Here's the drawing with two shaded views (mm, measured from the low corner). I have some questions. A direction names the side the tool comes from. Coordinates: 2 decimals unless noted, no trailing zeros. Order: outer loops, then holes, each group sorted by start corner. A loop starts at its lowest first (then second) coordinate and runs counter-clockwise, first axis right, second up. Notation, with made-up numbers: (-22.75, 20) -> (19.25, 20) arc R21 ccw to (19.25, 51) -> close; hole circle Ø6 at (-38, 88). An arc over 180 degrees is marked (long way). Return JSON: item names as keys, results as strings. Group by question number.
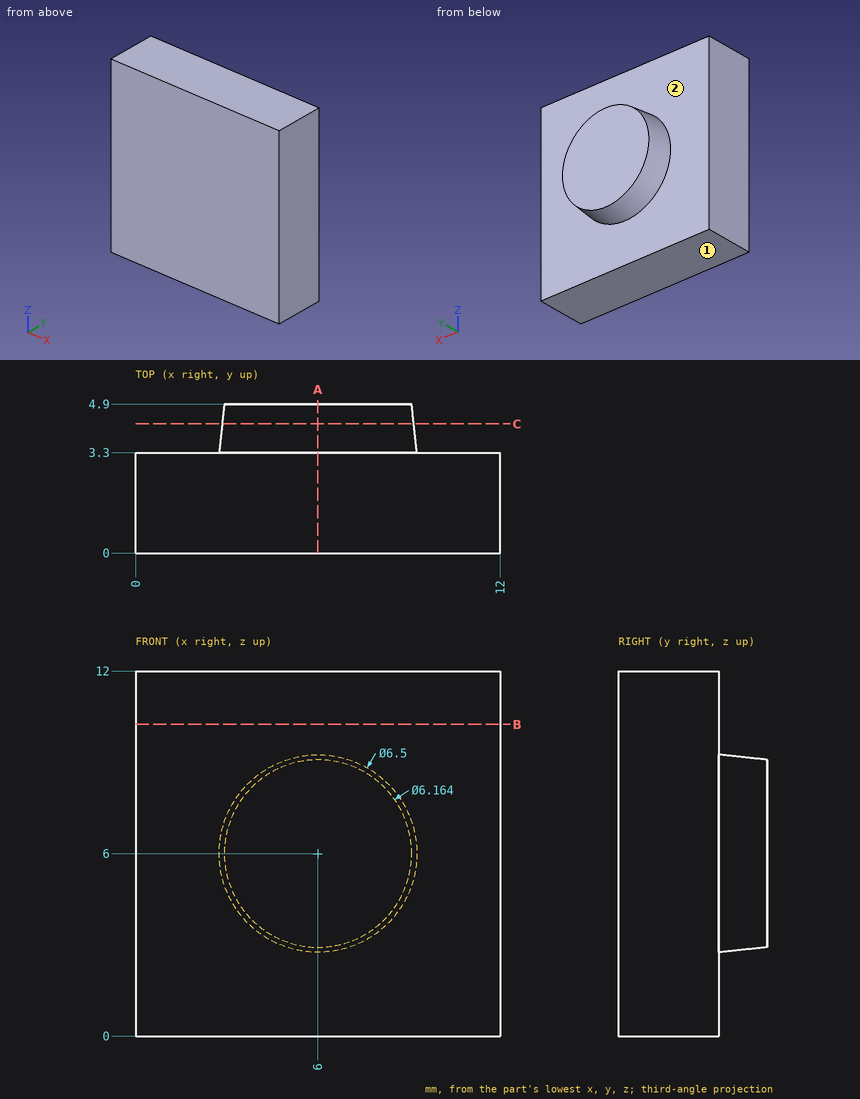
Q1. On a 3-axis mill with a long thin cutter (end or side, diameter ignored), from which of +Z, -Z, +X, -X, +Y, -Y can I reach the whole of each face in a straight line? I mean the marked faces 1 and 2. Say none if no direction works.
Q2. I want a section at B-B on z = 10.25. Please give me the cut outline in (x, y).
Q3. I want a section at C-C on y = 4.25. Please give me the cut outline in (x, z).
Q4. I need wall thicknesses on line 1 along Y through (x, z) = (4, 9); line 2 along Z through (x, y) = (3.25, 4.15) (1 decimal). Which ranges of each line are inside material? Lowest first, please. Write a range as from..to.
Q5. I want a section at A-A on x = 6. Please give me the cut outline in (y, z).
Response values:
{
 "1": {"face 1": "-Z, +X, -X, +Y, -Y", "face 2": "+Y"},
 "2": {"outline": "(0, 0) -> (12, 0) -> (12, 3.3) -> (0, 3.3) -> close"},
 "3": {"outline": "circle Ø6.3 at (6, 6)"},
 "4": {"line 1": "y = 0..3.3", "line 2": "z = 4.4..7.6"},
 "5": {"outline": "(0, 0) -> (3.3, 0) -> (3.3, 2.75) -> (4.9, 2.92) -> (4.9, 9.08) -> (3.3, 9.25) -> (3.3, 12) -> (0, 12) -> close"}
}
